from build123d import *

# Parameters (mm, degrees)
F0_W     = 80
F0_H     = 7.5
F0_R     = 2.25
F1_DEPTH = 2.5
F2_DEPTH = 5
F3_SIZE  = 1
F4_R     = 10
F5_R     = 5
F6_W     = 1
F6_H     = 7.5
F7_DEPTH = 0.5


with BuildPart() as f1:
    # F0 (on Top) → F1 (new body)
    with BuildSketch(Plane.XY):
        Rectangle(F0_W, F0_H)
        with BuildLine():
            Line((46.25, 10), (40, 3.75))
            Line((40, 3.75), (40, -3.75))
            Line((40, -3.75), (46.25, -10))
            Line((46.25, -10), (70, -10))
            ThreePointArc((70, -10), (80, 0), (70, 10))
            Line((70, 10), (46.25, 10))
        make_face()
        with Locations((70, 0)):
            Circle(F0_R, mode=Mode.SUBTRACT)
    extrude(amount=F1_DEPTH)

    # F0 (on Top) → F2 (join)
    with BuildSketch(Plane.XY):
        with BuildLine():
            Line((46.25, 10), (40, 3.75))
            Line((40, 3.75), (40, -3.75))
            Line((40, -3.75), (46.25, -10))
            Line((46.25, -10), (70, -10))
            ThreePointArc((70, -10), (80, 0), (70, 10))
            Line((70, 10), (46.25, 10))
        make_face()
        with Locations((70, 0)):
            Circle(F0_R, mode=Mode.SUBTRACT)
    extrude(amount=-F2_DEPTH)

    # F3
    f3_edges = [f1.edges().sort_by_distance(p)[0] for p in [
        (-40, -3.75, 1.25),
        (-40, 3.75, 1.25),
    ]]
    chamfer(f3_edges, length=F3_SIZE)

    # F4
    f4_edges = [f1.edges().sort_by_distance(p)[0] for p in [
        (40, -3.75, 1.25),
        (46.25, -10, -1.25),
        (46.25, 10, -1.25),
        (40, 3.75, 1.25),
    ]]
    fillet(f4_edges, radius=F4_R)

    # F5
    f5_edges = [f1.edges().sort_by_distance(p)[0] for p in [
        (40, -3.75, -2.5),
        (40, 3.75, -2.5),
    ]]
    fillet(f5_edges, radius=F5_R)

    # F6 (on face) → F7 (cut)
    with BuildSketch(Plane.XY.offset(2.5)):
        Rectangle(F6_W, F6_H)
    extrude(amount=-F7_DEPTH, mode=Mode.SUBTRACT)


solid = f1.part
Geometry check sheet. Reference: the model listing, model coordinates, mm. A direction names the side the tool comes from. Coordinates: 2 decimals unless noted, no trailing zeros. Order: outer loops, then holes, each group sorted by start corner. A loop starts at its lowest first (then second) coordinate and runs counter-clockwise, first axis right, second up. Notation, with made-up numbers: M 14,47.5 L 63,47.5 A19 ccw 63,60.5 Z; hole C -6.5,73 d11. An arc over 180 degrees is marked long. Use CSV: the item, a comma, the result in double quotes.
Item 1: Cross-section at B-B on z = -1.25. Record the cut outline in (x, y), then the cut area to 3 significant figures.
Returned:
outline,"M 40,-1.68 A5 ccw 41.46,-5.21 L 43.32,-7.07 A10 ccw 50.39,-10 L 70,-10 A10 ccw 70,10 L 50.39,10 A10 ccw 43.32,7.07 L 41.46,5.21 A5 ccw 40,1.68 Z; hole C 70,0 d4.5"
area,"697 mm2"
Item 2: Cross-section at D-D on y = 8.75. Record the cut outline in (x, z), then the cut area to 3 significant figures.
Returned:
outline,"M 45.55,-5 L 74.84,-5 L 74.84,2.5 L 45.55,2.5 Z"
area,"220 mm2"
Item 3: Cross-section at C-C on x = 28.5. Record the cut outline in (y, z).
Returned:
outline,"M -3.75,0 L 3.75,0 L 3.75,2.5 L -3.75,2.5 Z"
Item 4: Thickness scan on line 1 along Y through (x, z) = (70, 0); line 2 along Z through (x, y) = (-9.5, 1); line 3 along Y through (x, z) = (31.5, 0.75). Record the ranges inside material, lowest first.
Returned:
line 1,"y = -10 to -2.25, 2.25 to 10"
line 2,"z = 0 to 2.5"
line 3,"y = -3.75 to 3.75"
Item 5: Mould release check, pull along X, two halves, no side actions. Record for faces 6 (the cylindrical face through (40.39, -3.62, -2.54)), 7 (the cylindrical face through (72.08, -0.86, -1.3)), 8 (the cylindrical face through (80, 0, -1)): pulls with the +X half, pulls with the -X half, needs draft (parallel to the pull), parting line crosses it, or undercut.
Returned:
face 6,"pulls with the -X half"
face 7,"undercut"
face 8,"pulls with the +X half"
Item 6: Gauge pin test, flat ends, axial feed: pin 1 Ø1.2 at (x, z) = (0, 0.5) entering from +Y; pin 2 Ø3 at (x, z) = (43, 0) entering from +Y; pin 3 Ø1.5 at (y, z) = (-5, -3) entering from -X. Record the tip position at first contact, or that the pin passes through.
Returned:
pin 1,"stops at y = 3.75"
pin 2,"stops at y = 8.08"
pin 3,"stops at x = 40.71"
Item 7: Tool access check on faces 1 (the flat face through (-2, -3.75, 1)), 2 (the flat face through (40, 0, -2)), 3 (the flat face through (42.41, 6.16, -2.03)), 4 (the flat face through (-40, 0, 1)), 5 (the flat face through (60, -10, -1)). Record the directions out of +Z, -Z, +X, -X, +Y, -Y that give a thin tool (end or side, any length) a straight path to the whole face; none if there is none.
Returned:
face 1,"+Z, -Z, -X, -Y"
face 2,"-Z, -X, +Y, -Y"
face 3,"-Z, -X, +Y"
face 4,"+Z, -Z, -X, +Y, -Y"
face 5,"+Z, -Z, +X, -X, -Y"
Item 8: Cross-section at A-A on y = 0. Record the cut outline in (x, z), then the cut area to 3 significant figures.
Returned:
outline,"M -40,0 L 40,0 L 40,-5 L 67.75,-5 L 67.75,2.5 L 0.5,2.5 L 0.5,2 L -0.5,2 L -0.5,2.5 L -40,2.5 Z; M 72.25,-5 L 80,-5 L 80,2.5 L 72.25,2.5 Z"
area,"466 mm2"
